Here's how the part is built. I have some questions about the finished solid (model axes, mm). Coordinates: 2 decimals unless noted, no trailing zeros. Write each loop counter-clockwise with the first axis right and the second up, starting at its lowest first coordinate (ties: lowest second). Pieces come first, ordered by that corner, then holes. Notation, with made-up numbers: (21, 1.25) -> (51, 1.25) arc R28 cw to (51, 24.25) -> close; hole circle Ø9 at (35, 29.5). An arc over 180 degrees is marked (long way). Use a Markdown table: item, result. Add a question column.
Item 1: Will these pins go through, and if not, where does the flat tip stop? pin 1 Ø1.6 at (y, z) = (2, 38) entering from +X; pin 2 Ø1.6 at (y, z) = (1, -25.5) entering from -X; pin 3 Ø1.5 at (x, y) = (-12.5, 2) entering from -Z.
Item 2: Imagine slicing it at A-A, the plane x = 27.5. Write out the boundary of the cut face in (y, z) (3 decimals), and give its area (3 significant figures).
Item 3: If I drill on line 1 along X through (y, z) = (1.95, 41.91) (3 decimals); line 2 along X through (y, z) = (0.65, 39.5); line 3 along Z through (x, y) = (-3, 1), over which ranges is the centre line in solid material (lowest first)? Write a range as from..to.
Item 4: Imagine slicing it at C-C, the plane y = 2.5. Count the separate pieces of the cut face and the enclosed holes in it, and give its area (3 significant figures).
Item 5: Imagine slicing it at B-B, the plane z = 26. Write out the boundary of the cut face in (x, y) (3 decimals).
```python
from build123d import *

# Parameters (mm, degrees)
SKETCH1_W           = 80.01
SKETCH1_H           = 102.87
BOSS_EXTRUDE1_DEPTH = 3.175
SKETCH2_W           = 3.175
SKETCH2_H           = 6.35
CUT_EXTRUDE1_DEPTH  = 4.175
SKETCH3_W           = 6.35
SKETCH3_H           = 3.175
CUT_EXTRUDE2_DEPTH  = 4.175
SKETCH8_R           = 1.60809856
SKETCH8_R_2         = 1.608098511
SKETCH8_R_3         = 1.608098562
CUT_EXTRUDE3_DEPTH  = 4.175


with BuildPart() as part:
    # Sketch1 → Boss-Extrude1 (new body)
    with BuildSketch(Plane(origin=(0, 0, 0), x_dir=(1, 0, 0), z_dir=(0, 1, 0))):
        Rectangle(SKETCH1_W, SKETCH1_H)
    extrude(amount=BOSS_EXTRUDE1_DEPTH)

    # Sketch2 → Cut-Extrude1 (cut, through all)
    with BuildSketch(Plane(origin=(0, 3.175, 0), x_dir=(1, 0, 0), z_dir=(0, 1, 0))):
        with Locations((-38.4175, -38.1)):
            Rectangle(SKETCH2_W, SKETCH2_H)
        with Locations((-38.4175, -25.4)):
            Rectangle(SKETCH2_W, SKETCH2_H)
        with Locations((-38.4175, -12.7)):
            Rectangle(SKETCH2_W, SKETCH2_H)
        with Locations((-38.4175, 0)):
            Rectangle(SKETCH2_W, SKETCH2_H)
        with Locations((-38.4175, 12.7)):
            Rectangle(SKETCH2_W, SKETCH2_H)
        with Locations((-38.4175, 25.4)):
            Rectangle(SKETCH2_W, SKETCH2_H)
        with Locations((38.4175, 25.4)):
            Rectangle(SKETCH2_W, SKETCH2_H)
        with Locations((38.4175, 12.7)):
            Rectangle(SKETCH2_W, SKETCH2_H)
        with Locations((38.4175, 0)):
            Rectangle(SKETCH2_W, SKETCH2_H)
        with Locations((38.4175, -12.7)):
            Rectangle(SKETCH2_W, SKETCH2_H)
        with Locations((38.4175, -25.4)):
            Rectangle(SKETCH2_W, SKETCH2_H)
        with Locations((38.4175, -38.1)):
            Rectangle(SKETCH2_W, SKETCH2_H)
        with Locations((-38.4175, 38.1)):
            Rectangle(SKETCH2_W, SKETCH2_H)
        with Locations((38.4175, 38.1)):
            Rectangle(SKETCH2_W, SKETCH2_H)
    extrude(amount=-CUT_EXTRUDE1_DEPTH, mode=Mode.SUBTRACT)

    # Sketch3 → Cut-Extrude2 (cut, through all)
    with BuildSketch(Plane(origin=(0, 3.175, 0), x_dir=(1, 0, 0), z_dir=(0, 1, 0))):
        with Locations((25.4, 49.8475)):
            Rectangle(SKETCH3_W, SKETCH3_H)
        with Locations((12.7, 49.8475)):
            Rectangle(SKETCH3_W, SKETCH3_H)
        with Locations((0, 49.8475)):
            Rectangle(SKETCH3_W, SKETCH3_H)
        with Locations((-12.7, 49.8475)):
            Rectangle(SKETCH3_W, SKETCH3_H)
        with Locations((-12.7, -49.8475)):
            Rectangle(SKETCH3_W, SKETCH3_H)
        with Locations((0, -49.8475)):
            Rectangle(SKETCH3_W, SKETCH3_H)
        with Locations((12.7, -49.8475)):
            Rectangle(SKETCH3_W, SKETCH3_H)
        with Locations((25.4, -49.8475)):
            Rectangle(SKETCH3_W, SKETCH3_H)
        with Locations((-25.4, -49.8475)):
            Rectangle(SKETCH3_W, SKETCH3_H)
        with Locations((-25.4, 49.8475)):
            Rectangle(SKETCH3_W, SKETCH3_H)
    extrude(amount=-CUT_EXTRUDE2_DEPTH, mode=Mode.SUBTRACT)

    # Sketch8 → Cut-Extrude3 (cut, through all)
    with BuildSketch(Plane(origin=(-2.403797872, 3.175, 1.855162727), x_dir=(0, 0, 1), z_dir=(0, 1, 0))):
        with Locations((-10.706059909, 26.514695053)):
            Circle(SKETCH8_R)
        with Locations((-11.975611322, -21.707099309)):
            Circle(SKETCH8_R_2)
        with Locations((40.054837273, -16.628893673)):
            Circle(SKETCH8_R_3)
        with Locations((40.054837273, 11.280078142)):
            Circle(SKETCH8_R)
    extrude(amount=-CUT_EXTRUDE3_DEPTH, mode=Mode.SUBTRACT)


solid = part.part
```
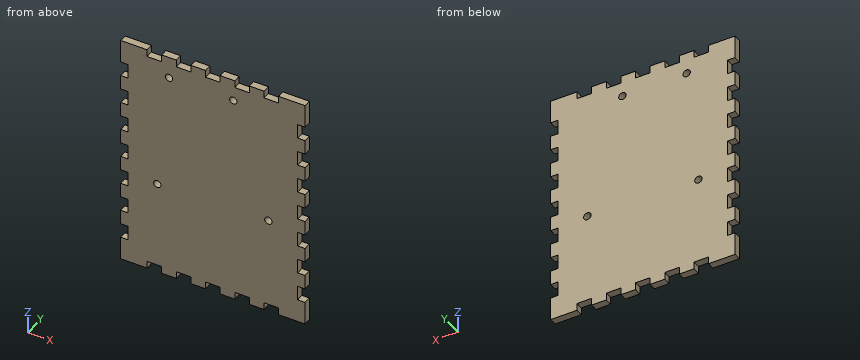
Ans:
| question | item | result |
|---|---|---|
| 1 | pin 1 | stops at x = 36.83 |
| 1 | pin 2 | stops at x = -36.83 |
| 1 | pin 3 | stops at z = -48.26 |
| 2 | outline | (0, -48.26) -> (3.175, -48.26) -> (3.175, 48.26) -> (0, 48.26) -> close |
| 2 | area | 306 mm^2 |
| 3 | line 1 | x = -40.005..-20.641, -17.425..7.268, 10.484..40.005 |
| 3 | line 2 | x = -36.83..36.83 |
| 3 | line 3 | z = -48.26..48.26 |
| 4 | separate pieces | 1 |
| 4 | enclosed holes | 4 |
| 4 | area | 7,710 mm^2 |
| 5 | outline | (-36.83, 0) -> (36.83, 0) -> (36.83, 3.175) -> (-36.83, 3.175) -> close |
